Geometry check sheet. Reference: the model listing, model coordinates, mm. A direction names the side the tool comes from. Coordinates: 2 decimals unless noted, no trailing zeros. Write each loop counter-clockwise with the first axis right and the second up, starting at its lowest first coordinate (ties: lowest second). Pieces come first, ordered by that corner, then holes. Notation, with made-up numbers: M 24,32.5 L 60,32.5 A20 cw 60,58.5 Z; hole C -30.5,-16.5 d2. An arc over 180 degrees is marked long. Put each result on its own line as item: value. Start each with the question number.
1) Set-up check for faces 4 (the flat face through (279, 18, 0.195)), 5 (the flat face through (317.5, 18, -49)), 6 (the cylindrical face through (-300.524, 19.012, 16.825)), 7 (the flat face through (-143, 18, -84.336)), 8 (the flat face through (172, 18, -24.805)): record each of +Z, -Z, +X, -X, +Y, -Y from which the full face is reachable in a straight line by a thin tool's end or side.
2) Gauge pin test, flat ends, axial feed: pin 1 (5 mm diameter, centred on y = 21, z = -109.5, fed in from -X); pin 2 (1 mm diameter, centred on y = 29.5, z = -66, fed in from -X); pin 3 (11 mm diameter, centred on x = -98.5, y = 13.5, fed in from -Z). Record the tip position at first contact, or that the pin passes through.
3) Cross-section at B-B on x = 240. Record the cut outline in (y, z).
4) Scan lines: line 1 along X through (y, z) = (8, -15); line 2 along Z through (x, y) = (201.5, 14.5); line 3 along Z through (x, y) = (-167, 6.5). Record each from-to range of solid material in increasing order.
5) Cross-section at A-A on y = 17. Count the separate pieces of the cut face and the enclosed holes in it, plus the area to 3 significant figures.
6) Mould release check, pull along Z, two halves, no side actions. Record for faces 1 (the flat face through (171, 18, -143.867)), 2 (the flat face through (4, 37.5, -56)), 3 (the cylindrical face through (-3.88, 18.49, 23.89)): released by +Z, released by -Z, zero draft, split by the parting line, or undercut.
from build123d import *

# Parameters (mm, degrees)
SKETCH1_R           = 19.84375
BOSS_EXTRUDE1_DEPTH = 37.5
FILLET1_R           = 59.53125
FILLET3_R           = 15.625


with BuildPart() as part:
    # Sketch1 → Boss-Extrude1 (new body)
    with BuildSketch(Plane(origin=(0, 0, 0), x_dir=(1, 0, 0), z_dir=(0, 1, 0))):
        Polygon((-317.5, -34.7265625), (-317.5, 84.3359375), (0, 84.3359375), (62.5, 143.8671875), (317.5, 143.8671875), (317.5, 24.8046875), (317.5, -0.1953125), (255, -0.1953125), (255, 24.8046875), (62.5, 24.8046875), (0, -34.7265625), align=None)
        with Locations(Location((-257.96875, 0, 0), (0, 0, 270))):
            Circle(SKETCH1_R, mode=Mode.SUBTRACT)
        with Locations(Location((-9.839661148, -4.9609375, 0), (0, 0, 270))):
            Circle(SKETCH1_R, mode=Mode.SUBTRACT)
    extrude(amount=BOSS_EXTRUDE1_DEPTH)

    # Fillet1
    fillet1_edges = [part.edges().sort_by_distance(p)[0] for p in [
        (62.5, 18.75, -24.8046875),
        (0, 18.75, 34.7265625),
        (0, 18.75, -84.3359375),
        (62.5, 18.75, -143.8671875),
        (317.5, 18.75, -143.8671875),
        (-317.5, 18.75, 34.7265625),
        (-317.5, 18.75, -84.3359375),
    ]]
    fillet(fillet1_edges, radius=FILLET1_R - 0.0001)  # a hair under: the kernel refuses the full size

    # Fillet3
    fillet3_edges = [part.edges().sort_by_distance(p)[0] for p in [
        (317.5, 18.75, 0.1953125),
    ]]
    fillet(fillet3_edges, radius=FILLET3_R)


solid = part.part
Answer key:
1. face 4: +Z, +X, +Y, -Y
1. face 5: +Z, -Z, +X, +Y, -Y
1. face 6: +Z, -X, +Y, -Y
1. face 7: -Z, -X, +Y, -Y
1. face 8: +Z, +Y, -Y
2. pin 1: stops at x = 23.79
2. pin 2: stops at x = -301.42
2. pin 3: stops at z = -84.34
3. outline: M 0,-143.87 L 37.5,-143.87 L 37.5,-24.8 L 0,-24.8 Z
4. line 1: x = -316.69 to -270.96, -244.98 to 53.58, 255 to 317.49
4. line 2: z = -143.87 to -24.8
4. line 3: z = -84.34 to 34.73
5. separate pieces: 1
5. enclosed holes: 2
5. area: 72,400 mm²
6. face 1: released by -Z
6. face 2: zero draft
6. face 3: undercut
